The listing builds one solid part. Answer for the finished solid, in the listing's coordinates (mm). Face numbers are marked on the shaded views. A direction names the side the tool comes from. Round coordinates to 2 decimals unless told otherwise and drop trailing zeros. Order: outer loops, then holes, each group sorted by start corner. A loop starts at its lowest first (then second) coordinate and runs counter-clockwise, first axis right, second up. Notation, with made-up numbers: M 32.5,73 L 50.5,73 A27 cw 50.5,108 Z; hole C 89.25,-27 d5. An arc over 180 degrees is marked long. Write item = value, one per line. Start each with the question number.
(1) For a pull along X with two mould halves and no side action, classify the marked faces 6, 7, 8 and 9 as released by +X, released by -X, zero draft, split by the parting line, or undercut.
(2) A cutting plane is placed at B-B, the plane z = 18.5. Determine the outline of the cut face in (x, y), and give its area (3 significant figures).
(3) Each of these flat-tipped pins is pushed along its axis until it touches: pin 1 (2.5 mm diameter, centred on x = 10, y = 13, fed in from +Z); pin 2 (1.2 mm diameter, centred on x = 4.5, z = 15, fed in from -Y); pin 3 (1.2 mm diameter, centred on y = 14.5, z = 15.5, fed in from -X). Where does it stop, or does it pass through?
(4) Straight lines are drawn through the part: probe 1 along X at (y, z) = (13, 19.35); probe 2 along Z at (x, y) = (0.85, 6); probe 3 along X at (y, z) = (0.85, 14.7). For each, find the intervals that lie inside material, in ascending order. Write a range as from..to.
(5) A cutting plane is placed at A-A, the plane x = 10. Determine the outline of the cut face in (y, z).
(6) Which of the six approach directions +Z, -Z, +X, -X, +Y, -Y give full straight-line access (tool end or side, diameter ignored) to the marked faces 1, 2, 3, 4 and 5?
from build123d import *

# Parameters (mm, degrees)
CYLINDER010_R     = 2
CYLINDER010_DEPTH = 2
CYLINDER009_R     = 2
CYLINDER009_DEPTH = 2
CYLINDER008_R     = 2
CYLINDER008_DEPTH = 2
CYLINDER007_R     = 2
CYLINDER007_DEPTH = 2
CYLINDER006_R     = 2
CYLINDER006_DEPTH = 2
ARRAY002_Y_COUNT  = 2
ARRAY002_Y_PITCH  = 9.5
ARRAY002_Z_COUNT  = 2
ARRAY002_Z_PITCH  = 9.5
CYLINDER005_R     = 2
CYLINDER005_DEPTH = 2
ARRAY001_X_COUNT  = 2
ARRAY001_X_PITCH  = 9.5
ARRAY001_Z_COUNT  = 2
ARRAY001_Z_PITCH  = 9.5
CYLINDER003_R     = 2
CYLINDER003_DEPTH = 2
CYLINDER002_R     = 2
CYLINDER002_DEPTH = 2
CYLINDER001_R     = 2
CYLINDER001_DEPTH = 2
CYLINDER_R        = 2
CYLINDER_DEPTH    = 2
ARRAY_X_COUNT     = 3
ARRAY_X_PITCH     = 5
ARRAY_Y_COUNT     = 2
ARRAY_Y_PITCH     = 6
BOX_W             = 20
BOX_H             = 20
BOX_DEPTH         = 20
FILLET_R          = 1


with BuildPart() as cilindre010:
    # Cylinder010 → Cylinder010 (new body)
    with BuildSketch(Plane(origin=(14, 20.1, 5), x_dir=(1, 0, 0), z_dir=(0, -1, 0))):
        Circle(CYLINDER010_R)
    extrude(amount=CYLINDER010_DEPTH)


with BuildPart() as cilindre009:
    # Cylinder009 → Cylinder009 (new body)
    with BuildSketch(Plane(origin=(6, 20.1, 15), x_dir=(1, 0, 0), z_dir=(0, -1, 0))):
        Circle(CYLINDER009_R)
    extrude(amount=CYLINDER009_DEPTH)


with BuildPart() as cilindre008:
    # Cylinder008 → Cylinder008 (new body)
    with BuildSketch(Plane(origin=(10, 10, -0.1), x_dir=(1, 0, 0), z_dir=(0, 0, 1))):
        Circle(CYLINDER008_R)
    extrude(amount=CYLINDER008_DEPTH)


with BuildPart() as cilindre007:
    # Cylinder007 → Cylinder007 (new body)
    with BuildSketch(Plane(origin=(18.1, 10, 10), x_dir=(0, 0, -1), z_dir=(1, 0, 0))):
        Circle(CYLINDER007_R)
    extrude(amount=CYLINDER007_DEPTH)


with BuildPart() as array002:
    # Cylinder006 → Cylinder006 (new body)
    with BuildSketch(Plane(origin=(0, 0, 0), x_dir=(0, 0, -1), z_dir=(1, 0, 0))):
        Circle(CYLINDER006_R)
    extrude(amount=CYLINDER006_DEPTH)

    # Array002 Y: Array002 ×2


with BuildPart() as array002_1:
    add(array002.part)
    with Locations(*[(0, i * ARRAY002_Y_PITCH, 0) for i in range(1, ARRAY002_Y_COUNT)]):
        add(array002.part)

    # Array002 Z: Array002 ×2


with BuildPart() as array002_2:
    add(array002_1.part)
    with Locations(*[(0, 0, i * ARRAY002_Z_PITCH) for i in range(1, ARRAY002_Z_COUNT)]):
        add(array002_1.part)


with BuildPart() as array002_3:
    # Array002 placement: moved
    add(array002_2.part.moved(Location((18.1, 5.3, 5.2))))


with BuildPart() as array001:
    # Cylinder005 → Cylinder005 (new body)
    with BuildSketch(Plane.XZ):
        Circle(CYLINDER005_R)
    extrude(amount=CYLINDER005_DEPTH)

    # Array001 X: Array001 ×2


with BuildPart() as array001_1:
    add(array001.part)
    with Locations(*[(i * ARRAY001_X_PITCH, 0, 0) for i in range(1, ARRAY001_X_COUNT)]):
        add(array001.part)

    # Array001 Z: Array001 ×2


with BuildPart() as array001_2:
    add(array001_1.part)
    with Locations(*[(0, 0, i * ARRAY001_Z_PITCH) for i in range(1, ARRAY001_Z_COUNT)]):
        add(array001_1.part)


with BuildPart() as array001_3:
    # Array001 placement: moved
    add(array001_2.part.moved(Location((5.3, 1.9, 5.2))))


with BuildPart() as cilindre003:
    # Cylinder003 → Cylinder003 (new body)
    with BuildSketch(Plane(origin=(0, 14, 15), x_dir=(0, 0, -1), z_dir=(1, 0, 0))):
        Circle(CYLINDER003_R)
    extrude(amount=CYLINDER003_DEPTH)


with BuildPart() as cilindre002:
    # Cylinder002 → Cylinder002 (new body)
    with BuildSketch(Plane(origin=(0, 10.1, 10), x_dir=(0, 0, -1), z_dir=(1, 0, 0))):
        Circle(CYLINDER002_R)
    extrude(amount=CYLINDER002_DEPTH)


with BuildPart() as cilindre001:
    # Cylinder001 → Cylinder001 (new body)
    with BuildSketch(Plane(origin=(1.9, 6, 5), x_dir=(0, 0, 1), z_dir=(-1, 0, 0))):
        Circle(CYLINDER001_R)
    extrude(amount=CYLINDER001_DEPTH)


with BuildPart() as array:
    # Cylinder → Cylinder (new body)
    with BuildSketch(Plane(origin=(5, 6.5, 18.1), x_dir=(1, 0, 0), z_dir=(0, 0, 1))):
        Circle(CYLINDER_R)
    extrude(amount=CYLINDER_DEPTH)

    # Array X: Array ×3


with BuildPart() as array_1:
    add(array.part)
    with Locations(*[(i * ARRAY_X_PITCH, 0, 0) for i in range(1, ARRAY_X_COUNT)]):
        add(array.part)

    # Array Y: Array ×2


with BuildPart() as array_2:
    add(array_1.part)
    with Locations(*[(0, i * ARRAY_Y_PITCH, 0) for i in range(1, ARRAY_Y_COUNT)]):
        add(array_1.part)


with BuildPart() as array_3:
    # Array placement: moved
    add(array_2.part.moved(Location((0, 0.5, 0))))


with BuildPart() as esfera:
    # Sphere → Sphere (revolve)
    with BuildSketch(Plane(origin=(10, 10, 10), x_dir=(1, 0, 0), z_dir=(0, -1, 0))):
        with BuildLine():
            ThreePointArc((0, -13.5), (13.5, 0), (0, 13.5))
            Line((0, 13.5), (0, -13.5))
        make_face()
    revolve(axis=Axis((10, 10, 10), (0, 0, 1)))


with BuildPart() as cut009:
    # Box → Box (new body)
    with BuildSketch(Plane.XY):
        with Locations((10, 10)):
            Rectangle(BOX_W, BOX_H)
    extrude(amount=BOX_DEPTH)

    # Fillet
    fillet_edges = [cut009.edges().sort_by_distance(p)[0] for p in [
        (0, 0, 10),
        (0, 10, 20),
        (0, 20, 10),
        (0, 10, 0),
        (20, 0, 10),
        (20, 10, 20),
        (20, 20, 10),
        (20, 10, 0),
        (10, 0, 0),
        (10, 0, 20),
        (10, 20, 0),
        (10, 20, 20),
    ]]
    fillet(fillet_edges, radius=FILLET_R)

    # Common: intersect Esfera
    add(esfera.part, mode=Mode.INTERSECT)

    # Cut: cut Array
    add(array_3.part, mode=Mode.SUBTRACT)

    # Cut001: cut Cilindre001
    add(cilindre001.part, mode=Mode.SUBTRACT)

    # Cut002: cut Cilindre002
    add(cilindre002.part, mode=Mode.SUBTRACT)

    # Cut003: cut Cilindre003
    add(cilindre003.part, mode=Mode.SUBTRACT)

    # Cut004: cut Array001
    add(array001_3.part, mode=Mode.SUBTRACT)

    # Cut005: cut Array002
    add(array002_3.part, mode=Mode.SUBTRACT)

    # Cut006: cut Cilindre007
    add(cilindre007.part, mode=Mode.SUBTRACT)

    # Cut007: cut Cilindre008
    add(cilindre008.part, mode=Mode.SUBTRACT)

    # Cut008: cut Cilindre009
    add(cilindre009.part, mode=Mode.SUBTRACT)

    # Cut009: cut Cilindre010
    add(cilindre010.part, mode=Mode.SUBTRACT)


solid = cut009.part
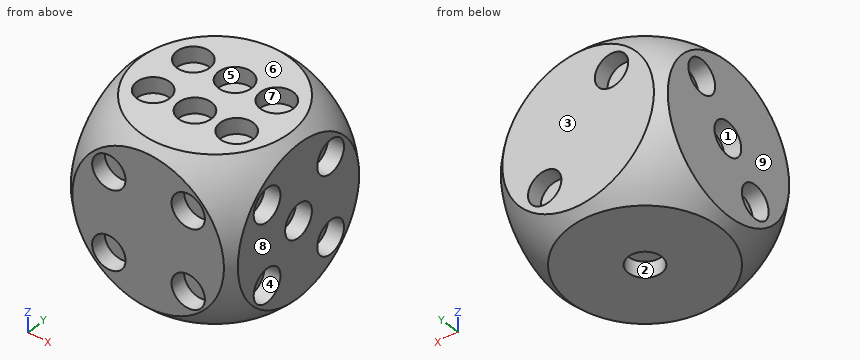
Reported:
q1.face_6 = zero draft
q1.face_7 = undercut
q1.face_8 = released by +X
q1.face_9 = released by -X
q2.outline = M 0,6.84 A10.49 ccw 6.84,0 L 13.16,0 A10.49 ccw 20,6.84 L 20,13.16 A10.49 ccw 13.16,20 L 6.84,20 A10.49 ccw 0,13.16 Z; hole C 5,7 d4; hole C 5,13 d4; hole C 10,7 d4; hole C 10,13 d4; hole C 15,7 d4; hole C 15,13 d4
q2.area = 262 mm²
q3.pin_1 = 18.1
q3.pin_2 = 1.9
q3.pin_3 = 2
q4.probe_1 = 0.74..3, 7..8, 12..13, 17..19.26
q4.probe_2 = 0.92..3, 7..19.08
q4.probe_3 = 1.26..3.3, 7.3..12.8, 16.8..18.74
q5.outline = M 0,0.93 A13.5 ccw 0.93,0 A1 ccw 1,0 L 8,0 L 8,1.9 L 12,1.9 L 12,0 L 19,0 A1 ccw 19.07,0 A13.5 ccw 20,0.93 A1 ccw 20,1 L 20,19 A1 ccw 20,19.07 A13.5 ccw 19.07,20 A1 ccw 19,20 L 15,20 L 15,18.1 L 11,18.1 L 11,20 L 9,20 L 9,18.1 L 5,18.1 L 5,20 L 1,20 A1 ccw 0.93,20 A13.5 ccw 0,19.07 A1 ccw 0,19 L 0,1 A1 ccw Z
q6.face_1 = -X
q6.face_2 = -Z
q6.face_3 = +Z, -Z, +X, -X, +Y
q6.face_4 = +X
q6.face_5 = +Z
